Can you work these out from the model? Positions are in its coordinate system, mm. Face numbers are marked on the shaded views. A direction names the side the tool comes from. Give positions to 0.01 mm unless a question says otherwise; leave off trailing zeros. Loops run counter-clockwise (first coordinate to the right, second up) from the corner with the lowest first, then second, coordinate; pieces in that order, holes last. Notation, with made-up numbers: (-27.75, -14.75) - (23.25, -14.75) arc R20 cw to (23.25, 17.25) - close; hole circle Ø2 at (-22.75, -34). An arc over 180 degrees is marked (long way). Use a Markdown table: item, result. Add a question column.
Autodesk Inventor part; units mm, degrees
ref_plane "YZ Plane" through (0, 0, 0) normal (1, 0, 0) x (0, 1, 0)
ref_plane "XZ Plane" through (0, 0, 0) normal (0, 1, 0) x (-1, 0, 0)
ref_plane "XY Plane" through (0, 0, 0) normal (0, 0, 1) x (1, 0, 0)
sketch "Sketch1" plane through (0, 0, 0) normal (1, 0, 0) x (0, 1, 0)
  line L0 (-20.6375, -12.7) -> (20.6375, -12.7) construction
  line L1 (20.6375, -12.7) -> (20.6375, 12.7) construction
  line L2 (20.6375, 12.7) -> (-20.6375, 12.7) construction
  line L3 (-20.6375, 12.7) -> (-20.6375, -12.7) construction
  line L4 (-20.6375, -12.7) -> (20.6375, 12.7) construction
  line L5 (20.6375, -12.7) -> (-20.6375, 12.7) construction
  circle A0 centre (-20.6375, 12.7) radius 4.7625 construction
  circle A1 centre (-20.6375, -12.7) radius 4.7625 construction
  circle A2 centre (20.6375, -12.7) radius 4.7625 construction
  circle A3 centre (20.6375, 12.7) radius 4.7625 construction
  line L6 (-25.4, -23.622) -> (25.4, -23.622)
  line L7 (25.4, -23.622) -> (25.4, 23.622)
  line L8 (25.4, 23.622) -> (-25.4, 23.622)
  line L9 (-25.4, 23.622) -> (-25.4, -23.622)
  line L10 (-25.4, -23.622) -> (25.4, 23.622) construction
  line L11 (25.4, -23.622) -> (-25.4, 23.622) construction
  line L12 (20.6375, -7.9375) -> (20.6375, 7.9375)
  line L13 (15.875, -12.7) -> (-15.875, -12.7)
  line L14 (-20.6375, 7.9375) -> (-20.6375, -7.9375)
  line L15 (-15.875, 12.7) -> (15.875, 12.7)
  arc A4 (15.875, 12.7) -> (20.6375, 7.9375) centre (20.6375, 12.7) ccw
  arc A5 (20.6375, -7.9375) -> (15.875, -12.7) centre (20.6375, -12.7) ccw
  arc A6 (-15.875, -12.7) -> (-20.6375, -7.9375) centre (-20.6375, -12.7) ccw
  arc A7 (-20.6375, 7.9375) -> (-15.875, 12.7) centre (-20.6375, 12.7) ccw
  line L16 (12.7, 18.161) -> (-12.7, 18.161) construction
  line L17 (12.7, 20.701) -> (-12.7, 20.701)
  line L18 (-12.7, 15.621) -> (12.7, 15.621)
  arc A8 (12.7, 15.621) -> (12.7, 20.701) centre (12.7, 18.161) ccw
  arc A9 (-12.7, 20.701) -> (-12.7, 15.621) centre (-12.7, 18.161) ccw
  line L19 (12.7, -18.161) -> (-12.7, -18.161) construction
  line L20 (12.7, -20.701) -> (-12.7, -20.701)
  line L21 (-12.7, -15.621) -> (12.7, -15.621)
  arc A10 (12.7, -20.701) -> (12.7, -15.621) centre (12.7, -18.161) ccw
  arc A11 (-12.7, -15.621) -> (-12.7, -20.701) centre (-12.7, -18.161) ccw
  line L22 (0, 23.622) -> (0, 12.7) construction
  line L23 (0, -12.7) -> (0, -23.622) construction
  point P0 (0, 0)
  point P1 (0, 18.161)
  point P2 (0, -18.161)
  point P3 (0, 18.161)
  point P4 (0, -18.161)
  dimension "d0" = 25.4
  dimension "d1" = 41.275
  dimension "d2" = 9.525
  dimension "d3" = 47.244
  dimension "d4" = 2.54
  dimension "d5" = 25.4
extrude "Extrusion1" add sketch "Sketch1" along normal blind 25.146
hole "Hole1" at (0, 20.6375, 12.7) at (0, 20.6375, -12.7) at (0, -20.6375, -12.7) at (0, -20.6375, 12.7) direction (1, 0, 0) diameter 5.1054 end through all
sketch "Sketch2" plane through (0, 25.4, 23.622) normal (0, 1, 0) x (1, 0, 0)
  point P0 (0, 23.622)
sketch "Sketch3" plane through (0, 25.4, 23.622) normal (0, 1, 0) x (1, 0, 0)
  line L0 (3.175, 15.6845) -> (21.9634, 15.6845)
  line L1 (21.9634, 15.6845) -> (21.9634, 31.5595)
  line L2 (21.9634, 31.5595) -> (3.175, 31.5595)
  line L3 (3.175, 31.5595) -> (3.175, 15.6845)
  line L4 (3.175, 15.6845) -> (21.9634, 31.5595) construction
  line L5 (21.9634, 15.6845) -> (3.175, 31.5595) construction
  line L6 (0, 47.244) -> (0, 0) construction
  line L7 (25.146, 47.244) -> (25.146, 0) construction
  line L8 (0, 15.6845) -> (25.146, 15.6845) construction
  point P0 (0, 23.622)
  point P1 (12.5692, 23.622)
  point P2 (21.9634, 23.622)
  point P3 (3.175, 23.622)
  point P4 (0, 23.622)
  point P5 (0, 23.622)
  point P6 (25.146, 23.622)
  dimension "d16" = 3.175
  dimension "d17" = 3.1826
extrude "Extrusion2" cut sketch "Sketch3" against normal through all
fillet "Fillet1" radius 3.175 4 edges at (12.573, 15.875, 12.7) (12.573, 15.875, -12.7) (12.573, -15.875, -12.7) (12.573, -15.875, 12.7)
fillet "Fillet2" radius 9.525 4 edges at (12.573, -25.4, -23.622) (12.573, -25.4, 23.622) (12.573, 25.4, 23.622) (12.573, 25.4, -23.622)
properties part number "EL2-022" material "ABS Plastic"
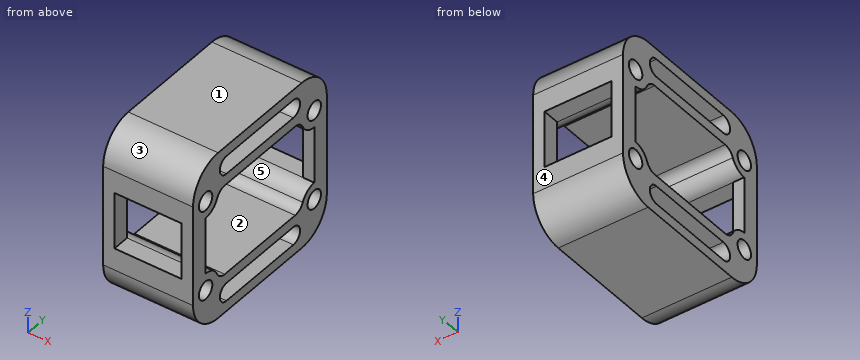
1. Suppose I cut it at B-B (z = -20). List the corners of the cut face in (x, y) for me.
2. Suppose I cut it at A-A (y = 10). List the corners of the cut face in (x, z) for me.
3. Please list where these lines run through material, in increasing order: line 1 along Z through (x, y) = (10.25, 11); line 2 along Z through (x, y) = (14.75, -21); line 3 along X through (y, z) = (-21, -4) (3 decimals). Write a range as [from, to].
4. Will this pin go through, and if not, where does the flat tip stop? P1, Ø1.4, axis at x = 14, y = 23.5, coming from the -Z side.
5. Suppose I cut it at C-C (x = 6.5). State how many separate pieces and enclosed holes the cut face has, and give its area (3 significant figures).
6. If we mould it in two halves opening along Y, with no side actions, what happens to the marked faces 1, 2 and 3? For each: released by +Y, released by -Y, zero draft, split by the parting line, or undercut.
7. On a 3-axis mill with a long thin cutter (end or side, diameter ignored), from which of +Z, -Z, +X, -X, +Y, -Y can I reach the whole of each face in a straight line? I mean the marked faces 4 and 5. Say none if no direction works.
Results below:
| question | item | result |
|---|---|---|
| 1 | outline | (0, -23.35) - (25.15, -23.35) - (25.15, -14.45) - (0, -14.45) - close; (0, 14.45) - (25.15, 14.45) - (25.15, 23.35) - (0, 23.35) - close |
| 2 | outline | (0, -23.62) - (25.15, -23.62) - (25.15, -20.7) - (0, -20.7) - close; (0, -15.62) - (25.15, -15.62) - (25.15, -12.7) - (0, -12.7) - close; (0, 12.7) - (25.15, 12.7) - (25.15, 15.62) - (0, 15.62) - close; (0, 20.7) - (25.15, 20.7) - (25.15, 23.62) - (0, 23.62) - close |
| 3 | line 1 | [-23.62, -20.7], [-15.62, -12.7], [12.7, 15.62], [20.7, 23.62] |
| 3 | line 2 | [-22.13, -15.23], [-10.17, -7.94], [7.94, 10.17], [15.23, 22.13] |
| 3 | line 3 | [0, 3.175], [21.963, 25.146] |
| 4 | P1 | z = -20.64 |
| 5 | separate pieces | 2 |
| 5 | enclosed holes | 6 |
| 5 | area | 817 mm² |
| 6 | face 1 | zero draft |
| 6 | face 2 | undercut |
| 6 | face 3 | released by -Y |
| 7 | face 4 | +Z, -Z, +X, -X, +Y |
| 7 | face 5 | +X, -X |
